from build123d import *

# Parameters (mm, degrees)
F1_DEPTH = 7
F2_R     = 1.25
F3_DEPTH = 25
F2_R_2   = 0.75
F4_DEPTH = 25
F5_DEPTH = 66
F6_DEPTH = 65.5


# Not quite as in the source:
# - a feature names something its author has since deleted; it is built from what else it names


with BuildPart() as f1:
    # F0 (on Right) → F1 (new body)
    with BuildSketch(Plane.YZ):
        Polygon((-25.6658861851, 12.3832505633), (-25.6658861851, -12.6167494367), (-8.6658861851, -12.6167494367), (-8.6658861851, -22.6167494367), (32.3341138149, -22.3259466936), (32.3341138149, -12.3259466936), (49.3341138149, -12.3259466936), (49.3341138149, 62.6740533064), (26.7576448203, 62.6740533064), (22.3341138149, 62.6740533064), (22.3341138149, 37.3832505633), (-0.6658861851, 37.3832505633), (-0.6658861851, 12.3832505633), align=None)
    extrude(amount=F1_DEPTH)



with BuildPart() as f3:
    # F2 (on Top) → F3 (new body)
    with BuildSketch(Plane.XY):
        with Locations((3.5, 25.5862374604)):
            Circle(F2_R)
    extrude(amount=F3_DEPTH)

    # F2 (on Top) → F4 (join)
    with BuildSketch(Plane.XY):
        with Locations((3.5, 25.5862374604)):
            Circle(F2_R)
    extrude(amount=F4_DEPTH)


with BuildPart() as f3b:
    # F2 (on Top) → F3, piece 2 (new body)
    with BuildSketch(Plane.XY):
        with Locations((3.5, 34.6862374604)):
            Circle(F2_R_2)
    extrude(amount=F3_DEPTH)

    # F2 (on Top) → F4, piece 2 (join)
    with BuildSketch(Plane.XY):
        with Locations((3.5, 34.6862374604)):
            Circle(F2_R_2)
    extrude(amount=F4_DEPTH)


with BuildPart() as f1_1:
    add(f1.part)

    add(f3.part)  # F5 merges F3
    # F2 (on Top) → F5 (join)
    with BuildSketch(Plane.XY):
        with Locations((3.5, 25.5862374604)):
            Circle(F2_R)
    extrude(amount=F5_DEPTH)


    add(f3b.part)  # F6 merges F3b
    # F2 (on Top) → F6 (join)
    with BuildSketch(Plane.XY):
        with Locations((3.5, 34.6862374604)):
            Circle(F2_R_2)
    extrude(amount=F6_DEPTH)


solid = f1_1.part
Here's how the part is built. I have some questions about the finished solid (model axes, mm). A direction names the side the tool comes from. Round coordinates to 2 decimals unless told otherwise and drop trailing zeros. Write each loop counter-clockwise with the first axis right and the second up, starting at its lowest first coordinate (ties: lowest second). Pieces come first, ordered by that corner, then holes.
1. I need wall thicknesses on L1, parallel to Z at x = 5, y = -12.5; L2, parallel to Z at x = 5, y = 34.5; L3, parallel to Y at x = 3.25, z = -18. Which ranges of each line are inside material? Lowest first, please.
2. Suppose I cut it at A-A (z = 54). List the corners of the cut face in (x, y) for me, and give its area (3 significant figures).
3. Will these pins go through, and if not, where does the flat tip stop? pin 1 Ø1 at (x, y) = (1.5, 11.5) entering from +Z; pin 2 Ø1.2 at (x, y) = (3.5, 34.5) entering from +Z; pin 3 Ø3.5 at (x, z) = (3.5, -18.5) entering from +Y.
4. Suppose I cut it at B-B (y = -16.5). List the corners of the cut face in (x, z) for me, and give its area (3 significant figures).
5. If we mould it in two halves opening along Y, with no side actions, what happens to faces 1 (the flat face through (3, -25.666, 0)), 2 (the cylindrical face through (4.17, 26.64, 64.31)), 3 (the flat face through (7, 20, 11))? For each: released by +Y, released by -Y, zero draft, split by the parting line, or undercut.
6. For faces 4 (the flat face through (3, 32.334, -17)), 5 (the flat face through (3, 22.334, 50)), 6 (the flat face through (3, -17, -12.617)), 7 (the flat face through (3, 26, 66)), which set-ups out of +Z, -Z, +X, -X, +Y, -Y let a thin tool reach every point of the face, with its end or its side?
Answer sheet:
1. L1: z = -12.62 to 12.38
1. L2: z = -12.33 to 62.67
1. L3: y = -8.67 to 32.33
2. outline: (0, 22.33) - (7, 22.33) - (7, 49.33) - (0, 49.33) - close
2. area: 189 mm2
3. pin 1: stops at z = 37.38
3. pin 2: stops at z = 65.5
3. pin 3: stops at y = 32.33
4. outline: (0, -12.62) - (7, -12.62) - (7, 12.38) - (0, 12.38) - close
4. area: 175 mm2
5. face 1: released by -Y
5. face 2: undercut
5. face 3: zero draft
6. face 4: -Z, +X, -X, +Y
6. face 5: +Z, +X, -X, -Y
6. face 6: -Z, +X, -X, -Y
6. face 7: +Z, +X, -X, +Y, -Y
